Part model, mm, in its own coordinate system. Face numbers are marked on the shaded views. A direction names the side the tool comes from. Round coordinates to 2 decimals unless told otherwise and drop trailing zeros. Order: outer loops, then holes, each group sorted by start corner. A loop starts at its lowest first (then second) coordinate and runs counter-clockwise, first axis right, second up. Notation, with made-up numbers: (33, -8.75) - (44, -8.75) arc R16 cw to (44, 8.25) - close; hole circle Ø7 at (31.5, 11). An arc over 180 degrees is marked (long way). Return JSON: item names as keys, results as strings. Group by question number.
Item 1: Tool access for the marked faces 4, 5 and 6: list every direction of +Z, -Z, +X, -X, +Y, -Y with a clear straight run to the whole face (end or side of a thin tool).
Item 2: Two-plate mould, pull along Y, no slides. Class the marked faces 1, 2 and 3: released by +Y, released by -Y, zero draft, split by the parting line, or undercut.
Item 3: Saw through at A-A on x = 4.5. List the corners of the cut face in (y, z).
Item 4: Probe probe 1 along X at (y, z) = (2, -1.75); probe 2 along Z at (x, y) = (5, 0); probe 3 along X at (y, z) = (-0.5, -2). List the from-to ranges inside material, lowest first.
Item 5: Drop flat-ended pins along their axis: pin 1 (1.5 mm diameter, centred on x = 7.5, z = -2, fed in from +Y); pin 2 (2 mm diameter, centred on x = -1, y = 3.5, fed in from +Z); pin 3 (1.5 mm diameter, centred on x = 2, y = 1.5, fed in from -Z). Give the stop position or say it passes through.
Autodesk Inventor part; units mm, degrees
ref_plane "Work Plane1" through (29, 0, 0) normal (0, -1, 0) x (1, 0, 0)
ref_plane "YZ Plane" through (0, 0, 0) normal (1, 0, 0) x (0, 1, 0)
ref_plane "XZ Plane" through (0, 0, 0) normal (0, 1, 0) x (-1, 0, 0)
sketch "Sketch1" plane through (0, 0, 0) normal (0, 0, 1) x (1, 0, 0)
  line L0 (0.2879, 0) -> (9.525, 0)
  line L1 (9.525, 0) -> (9.525, 2.413)
  line L2 (9.525, 2.413) -> (2.159, 2.413)
  line L3 (2.159, 2.413) -> (0.0422, 2.413)
  line L4 (0.0422, 2.413) -> (0, 2.413)
  line L5 (0, 2.413) -> (0, 4.5847)
  line L6 (0, 4.5847) -> (-2.5654, 4.5847)
  line L7 (-2.5654, 4.5847) -> (-2.5654, 1.8624)
  line L8 (-2.5654, 1.8624) -> (-0.7874, 1.8624)
  line L9 (-0.7874, 1.8624) -> (0.2879, 0)
  line L10 (-4.9835, 0) -> (11.9431, 0)
  line L11 (0, -0.9169) -> (0, 5.5016)
  line L12 (2.159, 2.413) -> (0, 2.413) construction
  dimension "d1" = 7.366
  dimension "d2" = 2.1168
  dimension "d3" = 2.5654
  dimension "d4" = 1.778
  dimension "d5" = 60
  dimension "d6" = 4.826
  dimension "d7" = 4.826
  dimension "d8" = 3.7248
  dimension "d9" = 9.1694
  dimension "d26" = 9.525
revolve "Body" add sketch "Sketch1" angle 360 about axis through (0.2879, 0, 0) along (1, 0, 0) contours L9 L11 L4 L3 L2 L1 L0 | L9 L8 L7 L6 L5 L11
sketch "Sketch2" plane through (-2.5654, 0, 0) normal (-1, 0, 0) x (0, 0, 1)
  circle A0 centre (0, 0) radius 1.8624
  line L0 (0, -6.4186) -> (0, 6.4186)
  line L1 (-6.4186, 0) -> (6.4186, 0)
  line L2 (1.8624, 0) -> (0.9312, -1.6129)
  line L3 (0.9312, -1.6129) -> (-0.9312, -1.6129)
  line L4 (-0.9312, -1.6129) -> (-1.8624, 0)
  line L5 (-1.8624, 0) -> (-0.9312, 1.6129)
  line L6 (-0.9312, 1.6129) -> (0.9312, 1.6129)
  line L7 (0.9312, 1.6129) -> (1.8624, 0)
extrude "Slot" add sketch "Sketch2" against normal up to next contours L7 A0 | A0 L2 | L6 L0 A0 | A0 L0 L3 | L0 L6 A0 | A0 L3 L0 | L4 A0 | A0 L5
fillet "Fillet1" radius 1.778 1 edges at (-2.5654, -4.5847, 0)
thread "Thread"
chamfer "Chamfer1" distance 0.6492 distance2 0.6492 1 edges at (9.525, -2.413, 0) measured on face at (9.525, -0.2686, 0.7084)
ref_plane "Work Plane1" through (29, 0, 0) normal (0, -1, 0) x (1, 0, 0)
fillet "Fillet2" radius 0.1 1 edges at (0, -2.413, 0)
equation "\"d30\" = R"
equation "\"d17\" = RR"
equation "\"d13\" = GEL"
equation "\"d15\" = -0.5 * SPD + 0.5 * GD"
equation "\"d16\" = GUL"
equation "\"d1\" = GEL"
equation "\"d3\" = KOH"
equation "\"d4\" = INTI"
equation "\"d6\" = GD"
equation "\"d7\" = BDM"
equation "\"d8\" = 1.1547 * SW"
equation "\"d9\" = KOD"
equation "\"d26\" = NLG"
equation "\"GD\" = NND"
equation "\"NLG\" = 9.525"
equation "\"GEL\" = 7.366"
equation "\"KOD\" = 9.1694"
equation "\"KOH\" = 2.5654"
equation "\"INTI\" = 1.778"
equation "\"GAL\" = 2.11668"
equation "\"GUL\" = 0.64922"
equation "\"BDM\" = NND"
equation "\"SW\" = 3.2258"
equation "\"RR\" = 1.778"
equation "\"SPD\" = GD1"
equation "\"R\" = 0.1"
equation "\"KR\" = 5.4102"
equation "\"GD1\" = 3.52755"
equation "\"THREADDIA\" = 4.826"
equation "\"FAWI\" = 45deg"
equation "\"KOH1\" = 1.778"
equation "\"NND\" = 4.826"
equation "\"TOA\" = 30deg"
equation "\"E0\" = 1.155 * SW"
properties part number "Unbrako - 10 x 3/8" material "Steel, Mild"
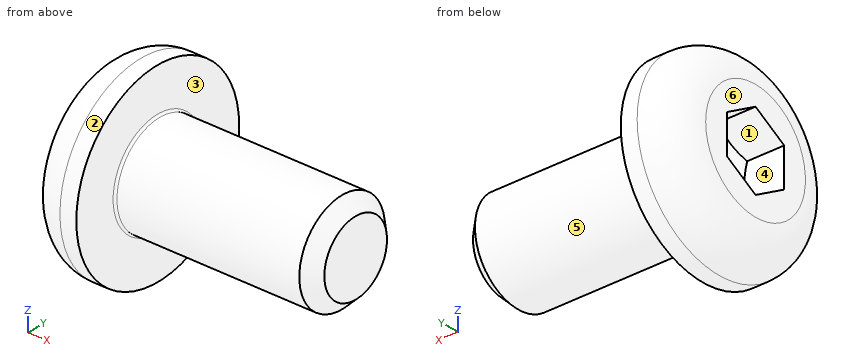
Filled in:
{
 "1": {"face 4": "-X", "face 5": "+X", "face 6": "+Z, -Z, -X, +Y, -Y"},
 "2": {"face 1": "undercut", "face 2": "split by the parting line", "face 3": "zero draft"},
 "3": {"outline": "circle Ø4.83 at (0, 0)"},
 "4": {"probe 1": "x = -2.57 to 0", "probe 2": "z = -2.41 to 2.41", "probe 3": "x = -2.57 to 9.23"},
 "5": {"pin 1": "stops at y = 2.06", "pin 2": "stops at z = 3.84", "pin 3": "stops at z = -2.29"}
}
